from build123d import *


with BuildPart() as part:
    # Sketch1 → Revolve1 (revolve)
    with BuildSketch(Plane.XY):
        with BuildLine():
            Line((0, 0), (0, 195))
            Line((0, 195), (-0.5, 195))
            ThreePointArc((-0.5, 195), (-2.621320344, 194.121320344), (-3.5, 192))
            Line((-3.5, 192), (-3.5, 159.571843893))
            ThreePointArc((-3.5, 159.571843893), (-3.607885473, 153.003545032), (-3.931425499, 146.442332412))
            Line((-3.931425499, 146.442332412), (-5.568574501, 121.557667588))
            ThreePointArc((-5.568574501, 121.557667588), (-5.892114527, 114.996454968), (-6, 108.428156107))
            Line((-6, 108.428156107), (-6, 0))
            Line((-6, 0), (0, 0))
        make_face()
    revolve(axis=Axis((0, 0, 0), (0, 1, 0)))


solid = part.part
Read the model definition and answer for the solid it produces. Units are mm, in the model's axes. A direction names the side the tool comes from. Give positions to 0.01 mm unless a question says otherwise; leave off trailing zeros. Loops run counter-clockwise (first coordinate to the right, second up) from the corner with the lowest first, then second, coordinate; pieces in that order, holes last. Notation, with made-up numbers: M 55.5,-38.75 L 65.5,-38.75 A25 ccw 65.5,0.25 Z; hole C 17,2.5 d1. An arc over 180 degrees is marked long. Write each question's results on one line, items separated by ' | '.
1. Given pin 1 (3 mm diameter, centred on x = 3.5, z = -1.5, fed in from +Y); pin 2 (5 mm diameter, centred on x = 2, y = 158.5, fed in from -Z); pin 3 (3 mm diameter, centred on y = 70, z = 2, fed in from +X), each flat-ended and moving along its own axis, determine where each tip first touches the part or whether it passes through.
Values:
pin 1: stops at y = 194.39 | pin 2: stops at z = -3.52 | pin 3: stops at x = 5.98
2. Straight lines are drawn through the part: line 1 (X direction, y = 44.5, z = 0.25); line 2 (X direction, y = 67.5, z = 4.5); line 3 (Z direction, x = -2.75, y = 124). For each, find the intervals that lie inside material, in ascending order. Write a range as [from, to].
Values:
line 1: x = [-5.99, 5.99] | line 2: x = [-3.97, 3.97] | line 3: z = [-4.66, 4.66]
3. Section B-B on y = 139.5 is taken. Give the vertices of the cut face in (x, z).
Values:
outline: C 0,0 d8.78
4. A tool of negligible diameter and unlimited length cuts with its end or side. For faces 1 (the face through (-3.233, 175.559, -1.341)), 2 (the face through (0, 0, 0)), from which of +Z, -Z, +X, -X, +Y, -Y can it reach the whole face along a straight path? Write none if from no direction.
Values:
face 1: +Y | face 2: +Z, -Z, +X, -X, -Y
5. Section A-A on y = 42.5 is taken. Give the vertices of the cut face in (x, z).
Values:
outline: C 0,0 d12
